from build123d import *

# Parameters (mm, degrees)
SKETCH_W      = 234
SKETCH_H      = 130
PAD_DEPTH     = 5
SKETCH002_R   = 2.4
SKETCH002_R_2 = 5
POCKET_DEPTH  = 5


with BuildPart() as part:
    # Sketch → Pad (new body)
    with BuildSketch(Plane.XZ):
        Rectangle(SKETCH_W, SKETCH_H)
    extrude(amount=PAD_DEPTH)

    # Sketch002 → Pocket (cut)
    with BuildSketch(Plane.XZ.offset(5)):
        with Locations((-94, 42)):
            Circle(SKETCH002_R)
        with Locations((-10, 42)):
            Circle(SKETCH002_R)
        with Locations((-10, -42)):
            Circle(SKETCH002_R)
        with Locations((-94, -42)):
            Circle(SKETCH002_R)
        with Locations((94, 42)):
            Circle(SKETCH002_R)
        with Locations((10, 42)):
            Circle(SKETCH002_R)
        with Locations((94, -42)):
            Circle(SKETCH002_R)
        with Locations((10, -42)):
            Circle(SKETCH002_R)
        with Locations((32, 30)):
            Circle(SKETCH002_R_2)
        with Locations((52, 30)):
            Circle(SKETCH002_R_2)
        with Locations((72, 30)):
            Circle(SKETCH002_R_2)
        with Locations((32, 10)):
            Circle(SKETCH002_R_2)
        with Locations((52, 10)):
            Circle(SKETCH002_R_2)
        with Locations((72, 10)):
            Circle(SKETCH002_R_2)
        with Locations((72, -10)):
            Circle(SKETCH002_R_2)
        with Locations((52, -10)):
            Circle(SKETCH002_R_2)
        with Locations((32, -10)):
            Circle(SKETCH002_R_2)
        with Locations((42, -30)):
            Circle(SKETCH002_R_2)
        with Locations((62, -30)):
            Circle(SKETCH002_R_2)
        with BuildLine():
            ThreePointArc((-93.291646, 13), (-94.291646, 12), (-93.291646, 11))
            Line((-93.291646, 11), (-10.708354, 11))
            ThreePointArc((-10.708354, 11), (-9.708354, 12), (-10.708354, 13))
            Line((-93.291646, 13), (-10.708354, 13))
        make_face()
        with BuildLine():
            ThreePointArc((-75.515952, 37), (-76.515952, 36), (-75.515952, 35))
            Line((-75.515952, 35), (-28.484048, 35))
            ThreePointArc((-28.484048, 35), (-27.484048, 36), (-28.484048, 37))
            Line((-75.515952, 37), (-28.484048, 37))
        make_face()
        with BuildLine():
            ThreePointArc((-82.805844, 31), (-83.805844, 30), (-82.805844, 29))
            Line((-82.805844, 29), (-21.194156, 29))
            ThreePointArc((-21.194156, 29), (-20.194156, 30), (-21.194156, 31))
            Line((-82.805844, 31), (-21.194156, 31))
        make_face()
        with BuildLine():
            ThreePointArc((-87.679126, 25), (-88.679126, 24), (-87.679126, 23))
            Line((-87.679126, 23), (-16.320874, 23))
            ThreePointArc((-16.320874, 23), (-15.320874, 24), (-16.320874, 25))
            Line((-87.679126, 25), (-16.320874, 25))
        make_face()
        with BuildLine():
            ThreePointArc((-91.051248, 19), (-92.051248, 18), (-91.051248, 17))
            Line((-91.051248, 17), (-12.948752, 17))
            ThreePointArc((-12.948752, 17), (-11.948752, 18), (-12.948752, 19))
            Line((-91.051248, 19), (-12.948752, 19))
        make_face()
        with BuildLine():
            ThreePointArc((-95, 1), (-96, 0), (-95, -1))
            Line((-95, -1), (-9, -1))
            ThreePointArc((-9, -1), (-8, 0), (-9, 1))
            Line((-95, 1), (-9, 1))
        make_face()
        with BuildLine():
            ThreePointArc((-94.579338, 7), (-95.579338, 6), (-94.579338, 5))
            Line((-94.579338, 5), (-9.420662, 5))
            ThreePointArc((-9.420662, 5), (-8.420662, 6), (-9.420662, 7))
            Line((-94.579338, 7), (-9.420662, 7))
        make_face()
        with BuildLine():
            ThreePointArc((-61.219544, 43), (-62.219544, 42), (-61.219544, 41))
            Line((-61.219544, 41), (-42.780456, 41))
            ThreePointArc((-42.780456, 41), (-41.780456, 42), (-42.780456, 43))
            Line((-61.219544, 43), (-42.780456, 43))
        make_face()
        with BuildLine():
            ThreePointArc((-61.219544, -41), (-62.219544, -42), (-61.219544, -43))
            Line((-61.219544, -43), (-42.780456, -43))
            ThreePointArc((-42.780456, -43), (-41.780456, -42), (-42.780456, -41))
            Line((-61.219544, -41), (-42.780456, -41))
        make_face()
        with BuildLine():
            ThreePointArc((-75.515952, -35), (-76.515952, -36), (-75.515952, -37))
            Line((-75.515952, -37), (-28.484048, -37))
            ThreePointArc((-28.484048, -37), (-27.484048, -36), (-28.484048, -35))
            Line((-75.515952, -35), (-28.484048, -35))
        make_face()
        with BuildLine():
            ThreePointArc((-82.805844, -29), (-83.805844, -30), (-82.805844, -31))
            Line((-82.805844, -31), (-21.194156, -31))
            ThreePointArc((-21.194156, -31), (-20.194156, -30), (-21.194156, -29))
            Line((-82.805844, -29), (-21.194156, -29))
        make_face()
        with BuildLine():
            ThreePointArc((-87.679126, -23), (-88.679126, -24), (-87.679126, -25))
            Line((-87.679126, -25), (-16.320874, -25))
            ThreePointArc((-16.320874, -25), (-15.320874, -24), (-16.320874, -23))
            Line((-87.679126, -23), (-16.320874, -23))
        make_face()
        with BuildLine():
            ThreePointArc((-91.051248, -17), (-92.051248, -18), (-91.051248, -19))
            Line((-91.051248, -19), (-12.948752, -19))
            ThreePointArc((-12.948752, -19), (-11.948752, -18), (-12.948752, -17))
            Line((-91.051248, -17), (-12.948752, -17))
        make_face()
        with BuildLine():
            ThreePointArc((-93.291646, -11), (-94.291646, -12), (-93.291646, -13))
            Line((-93.291646, -13), (-10.708354, -13))
            ThreePointArc((-10.708354, -13), (-9.708354, -12), (-10.708354, -11))
            Line((-93.291646, -11), (-10.708354, -11))
        make_face()
        with BuildLine():
            ThreePointArc((-94.579338, -5), (-95.579338, -6), (-94.579338, -7))
            Line((-94.579338, -7), (-9.420662, -7))
            ThreePointArc((-9.420662, -7), (-8.420662, -6), (-9.420662, -5))
            Line((-94.579338, -5), (-9.420662, -5))
        make_face()
    extrude(amount=-POCKET_DEPTH, mode=Mode.SUBTRACT)


solid = part.part
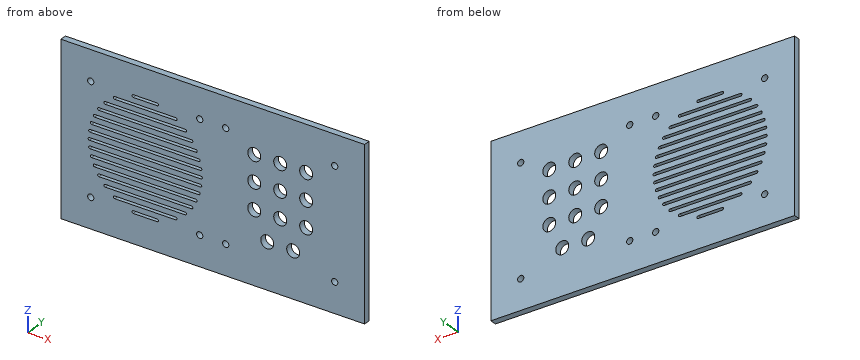
Read the model definition and answer for the solid it produces. Units are mm, in the model's axes. Round coordinates to 2 decimals unless told otherwise and drop trailing zeros. Write each loop counter-clockwise with the first axis right and the second up, starting at its lowest first coordinate (ties: lowest second). Pieces come first, ordered by that corner, then holes. Notation, with made-up numbers: (24, -10) - (77, -10) arc R25 cw to (77, 26) - close; hole circle Ø10 at (44, 48.5). An arc over 180 degrees is marked (long way). Use a Markdown table: item, result.
(1) The part is cut by section B-B (y = -1.7). State how many separate pieces and enclosed holes the cut face has, then the cut area to 3 significant figures.
Reported:
| item | result |
|---|---|
| separate pieces | 1 |
| enclosed holes | 34 |
| area | 27,400 mm2 |
(2) The part is cut by section A-A (x = 32). Write down the section's boundary in (y, z).
Reported:
| item | result |
|---|---|
| outline | (-5, -65) - (0, -65) - (0, -15) - (-5, -15) - close; (-5, -5) - (0, -5) - (0, 5) - (-5, 5) - close; (-5, 15) - (0, 15) - (0, 25) - (-5, 25) - close; (-5, 35) - (0, 35) - (0, 65) - (-5, 65) - close |
(3) Straight lines are drawn through the part: line 1 along Z through (x, y) = (94, -3.95); line 2 along Z through (x, y) = (72, -3.75); line 3 along X through (y, z) = (-1.9, 14.5). For each, find the intervals that lie inside material, in ascending order. Write a range as [from, to].
Reported:
| item | result |
|---|---|
| line 1 | [-65, -44.4], [-39.6, 39.6], [44.4, 65] |
| line 2 | [-65, -15], [-5, 5], [15, 25], [35, 65] |
| line 3 | [-117, 29.82], [34.18, 49.82], [54.18, 69.82], [74.18, 117] |
